Design review of the part built by this model. Coordinates are the model's own, in mm. Face numbers are marked on the shaded views. A direction names the side the tool comes from. Give positions to 0.01 mm unless a question says otherwise; leave off trailing zeros. Loops run counter-clockwise (first coordinate to the right, second up) from the corner with the lowest first, then second, coordinate; pieces in that order, holes last. Notation, with made-up numbers: M 7,-37 L 48,-37 A22 ccw 48,-27 Z; hole C 25.25,37 d3. An arc over 180 degrees is marked long. Use CSV: the item, a comma, the result in double quotes.
from build123d import *

# Parameters (mm, degrees)
SKETCH_1_R          = 2.75
EXTRUDE_1_DEPTH     = 2.5
SKETCH_2_R          = 12
EXTRUDE_2_DEPTH     = 11.9
CUT_EXTRUDE_1_DEPTH = 11.9
SKETCH_4_R          = 1.5
CUT_EXTRUDE_2_DEPTH = 38.043126228


with BuildPart() as part:
    # 草图1 → 凸台-拉伸1 (new, symmetric)
    with BuildSketch(Plane.XY):
        with BuildLine():
            Line((-25, 0), (25, 0))
            ThreePointArc((25, 0), (30.012842263, -12), (25, -24))
            Line((25, -24), (-25, -24))
            ThreePointArc((-25, -24), (-29.987157737, -12), (-25, 0))
        make_face()
        with Locations((-22.5, -12)):
            Circle(SKETCH_1_R, mode=Mode.SUBTRACT)
        with Locations((22.5, -12)):
            Circle(SKETCH_1_R, mode=Mode.SUBTRACT)
    extrude(amount=EXTRUDE_1_DEPTH, both=True)

    # 草图2 → 凸台-拉伸2 (add)
    with BuildSketch(Plane.XY.offset(2.5)):
        with Locations(Location((0, -12, 0), (0, 0, 270))):
            Circle(SKETCH_2_R)
    extrude(amount=EXTRUDE_2_DEPTH)

    # 草图3 → 切除-拉伸1 (cut)
    with BuildSketch(Plane.XY.offset(14.4)):
        with BuildLine():
            Line((-3.082207001, -7.75), (3.082207001, -7.75))
            ThreePointArc((3.082207001, -7.75), (0, -17.25), (-3.082207001, -7.75))
        make_face()
    extrude(amount=-CUT_EXTRUDE_1_DEPTH, mode=Mode.SUBTRACT)

    # 草图4 → 切除-拉伸2 (cut, through all)
    with BuildSketch(Plane.XZ.offset(7.75)):
        with Locations(Location((0, 11.4, 0), (0, 0, 270))):
            Circle(SKETCH_4_R)
        with Locations(Location((0, 5.4, 0), (0, 0, 270))):
            Circle(SKETCH_4_R)
    extrude(amount=-CUT_EXTRUDE_2_DEPTH, mode=Mode.SUBTRACT)


solid = part.part
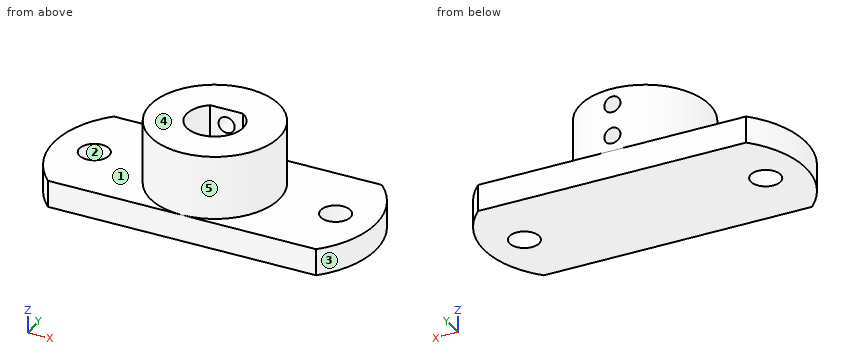
(1) Machinability: for the marked faces 4 and 5, which of the approach directions +Z, -Z, +X, -X, +Y, -Y give a long, thin tool a straight path to every point of the face, cutting with its end or side? Answer none if there is none.
A:
face 4,"+Z, +X, -X, +Y, -Y"
face 5,"+Z"
(2) The part is to be moulded in two halves that separate along X. For the marked faces 1, 2 and 3, say which applies: released by +X, released by -X, zero draft, split by the parting line, or undercut.
A:
face 1,"zero draft"
face 2,"undercut"
face 3,"released by +X"
(3) We need section C-C on y = -16. State the section outline as (x, z) points, then the cut area to 3 significant figures.
A:
outline,"M -29.51,-2.5 L 29.53,-2.5 L 29.53,2.5 L 11.31,2.5 L 11.31,14.4 L 3.4,14.4 L 3.4,2.5 L -3.4,2.5 L -3.4,14.4 L -11.31,14.4 L -11.31,2.5 L -29.51,2.5 Z"
area,"484 mm²"
(4) Clearance check with flat-ended pins moving along their axes: P1, Ø1, axis at y = -21, z = 12, coming from the -X side; P2, Ø1.8, axis at x = 0, z = 11.4, coming from the +Y side; P3, Ø2.5, axis at x = 0, z = 5.4, coming from the +Y side. State where each tip first meets the part, or that it passes through.
A:
P1,"x = -8.47"
P2,"y = -17.17"
P3,"y = -17.1"
(5) We need section A-A on x = -22.5. State the section outline as (y, z) points, then the cut area to 3 significant figures.
A:
outline,"M -24,-2.5 L -14.75,-2.5 L -14.75,2.5 L -24,2.5 Z; M -9.25,-2.5 L 0,-2.5 L 0,2.5 L -9.25,2.5 Z"
area,"92.5 mm²"
(6) Wall thickness on line 1 along Z through (x, y) = (0, -2); line 2 along X through (y, z) = (-12, 7.5); line 3 along Y through (x, z) = (-22.5, -0.15): over which ranges is each line inside the solid? List them lowest first. Write a range as [from, to].
A:
line 1,"[-2.5, 3.9], [6.9, 9.9], [12.9, 14.4]"
line 2,"[-12, -5.25], [5.25, 12]"
line 3,"[-24, -14.75], [-9.25, 0]"
(7) We need section D-D on x = -6.5. State the section outline as (y, z) points, then the cut area to 3 significant figures.
A:
outline,"M -24,-2.5 L 0,-2.5 L 0,2.5 L -1.91,2.5 L -1.91,14.4 L -22.09,14.4 L -22.09,2.5 L -24,2.5 Z"
area,"360 mm²"
(8) We need section B-B on z = -1. State the section outline as (x, y) points.
A:
outline,"M -25,-24 L 25,-24 A16.87 ccw 25,0 L -25,0 A16.93 ccw Z; hole C -22.5,-12 d5.5; hole C 22.5,-12 d5.5"
